The listing builds one solid part. Answer for the finished solid, in the listing's coordinates (mm). Coordinates: 2 decimals unless noted, no trailing zeros. One line per question, with ' | ' between items.
from build123d import *

# Parameters (mm, degrees)
SKETCH1_R               = 125
SKETCH1_R_2             = 32
BOSS_EXTRUDE1_DEPTH     = 4
CUT_EXTRUDE1_REACH      = 178.958
SKETCH2_R               = 4.5
CIRPATTERN2_COUNT       = 5
FILL_START              = -4
FILL_PATTERN1_OUTLINE_R = 4.5
FILL_PATTERN1_DEPTH     = 8
FILLET1_R               = 6.5


# Read off the part's stored shape, not the designer's step: Fill Pattern1
with BuildPart() as part:
    # Sketch1 → Boss-Extrude1 (new, symmetric)
    with BuildSketch(Plane.XY):
        Circle(SKETCH1_R)
        Circle(SKETCH1_R_2, mode=Mode.SUBTRACT)
    extrude(amount=BOSS_EXTRUDE1_DEPTH, both=True)

    # Sketch2 → Cut-Extrude1 (cut, up to next)
    with BuildSketch(Plane.XY.offset(4), mode=Mode.PRIVATE) as cut_extrude1_sk1:
        with BuildLine():
            ThreePointArc((-9.355894551, 30.601752191), (0, 32), (9.355894551, 30.601752191))
            Line((9.355894551, 30.601752191), (19.588904216, 64.07241865))
            ThreePointArc((19.588904216, 64.07241865), (0, 67), (-19.588904216, 64.07241865))
            Line((-19.588904216, 64.07241865), (-9.355894551, 30.601752191))
        make_face()
    cut_extrude1_tool1 = extrude(cut_extrude1_sk1.sketch, amount=-CUT_EXTRUDE1_REACH, mode=Mode.PRIVATE) & part.part
    # Sketch2 → Cut-Extrude1 (cut, up to next)
    with BuildSketch(Plane.XY.offset(4), mode=Mode.PRIVATE) as cut_extrude1_sk2:
        with Locations((-26.450336353, 36.405764747)):
            Circle(SKETCH2_R)
    cut_extrude1_tool2 = extrude(cut_extrude1_sk2.sketch, amount=-CUT_EXTRUDE1_REACH, mode=Mode.PRIVATE) & part.part
    cut_extrude1_1 = cut_extrude1_tool1.solids().sort_by_distance((0, 50.80907, 4))[0]
    add(cut_extrude1_1, mode=Mode.SUBTRACT)
    cut_extrude1_2 = cut_extrude1_tool2.solids().sort_by_distance((-26.450336, 36.405765, 4))[0]
    add(cut_extrude1_2, mode=Mode.SUBTRACT)
    cut_extrude1 = cut_extrude1_1 + cut_extrude1_2  # Cut-Extrude1 as one shape, for the pattern or mirror that repeats it

    # CirPattern2: Cut-Extrude1 ×5 about axis
    cirpattern2_axis = Axis((0, 0, 0), (0, 0, 1))
    for i in range(1, CIRPATTERN2_COUNT):
        add(cut_extrude1.rotate(cirpattern2_axis, i * 360 / CIRPATTERN2_COUNT), mode=Mode.SUBTRACT)

    # Fill Pattern1 outline → Fill Pattern1 (cut)
    with BuildSketch(Plane.XY.offset(FILL_START)):
        with Locations((-99.984772584, 1.745240337)):
            Circle(FILL_PATTERN1_OUTLINE_R)
        with Locations((-97.277590889, -23.174790656)):
            Circle(FILL_PATTERN1_OUTLINE_R)
        with Locations((-88.45810059, -46.638664341)):
            Circle(FILL_PATTERN1_OUTLINE_R)
        with Locations((-74.080462697, -67.172059239)):
            Circle(FILL_PATTERN1_OUTLINE_R)
        with Locations((-55.048077077, -83.484786633)):
            Circle(FILL_PATTERN1_OUTLINE_R)
        with Locations((-32.556818514, -94.551857867)):
            Circle(FILL_PATTERN1_OUTLINE_R)
        with Locations((-8.019895501, -99.677888152)):
            Circle(FILL_PATTERN1_OUTLINE_R)
        with Locations((17.020946849, -98.540790155)):
            Circle(FILL_PATTERN1_OUTLINE_R)
        with Locations((40.992300316, -91.212011924)):
            Circle(FILL_PATTERN1_OUTLINE_R)
        with Locations((62.387956603, -78.152047549)):
            Circle(FILL_PATTERN1_OUTLINE_R)
        with Locations((79.863547937, -60.181502622)):
            Circle(FILL_PATTERN1_OUTLINE_R)
        with Locations((92.321018643, -38.429532573)):
            Circle(FILL_PATTERN1_OUTLINE_R)
        with Locations((98.977620023, -14.262893677)):
            Circle(FILL_PATTERN1_OUTLINE_R)
        with Locations((99.415093329, 10.799935264)):
            Circle(FILL_PATTERN1_OUTLINE_R)
        with Locations((93.605950506, 35.184164534)):
            Circle(FILL_PATTERN1_OUTLINE_R)
        with Locations((81.915201361, 57.357643328)):
            Circle(FILL_PATTERN1_OUTLINE_R)
        with Locations((65.077418659, 75.927130427)):
            Circle(FILL_PATTERN1_OUTLINE_R)
        with Locations((44.150582211, 89.725836661)):
            Circle(FILL_PATTERN1_OUTLINE_R)
        with Locations((20.449602116, 97.886738569)):
            Circle(FILL_PATTERN1_OUTLINE_R)
        with Locations((-4.536301881, 99.897056672)):
            Circle(FILL_PATTERN1_OUTLINE_R)
        with Locations((-29.23717354, 95.63047529)):
            Circle(FILL_PATTERN1_OUTLINE_R)
        with Locations((-52.100966252, 85.355079421)):
            Circle(FILL_PATTERN1_OUTLINE_R)
        with Locations((-71.691063833, 69.716509979)):
            Circle(FILL_PATTERN1_OUTLINE_R)
        with Locations((-86.776548405, 49.697395796)):
            Circle(FILL_PATTERN1_OUTLINE_R)
        with Locations((-96.409543491, 26.555611442)):
            Circle(FILL_PATTERN1_OUTLINE_R)
    extrude(amount=FILL_PATTERN1_DEPTH, mode=Mode.SUBTRACT)

    # Fillet1
    fillet1_edges = [part.edges().sort_by_distance(p)[0] for p in [
        (19.588904216, 64.07241865, 0),
        (9.355894551, 30.601752191, 0),
        (-9.355894551, 30.601752191, 0),
        (-19.588904216, 64.07241865, 0),
        (-53.508579173, -40.321606551, 0),
        (-25.556336322, -19.258080741, 0),
        (-10.418180943, -30.256594419, 0),
        (-21.813066349, -63.349744565, 0),
        (21.813066349, -63.349744565, 0),
        (10.418180943, -30.256594419, 0),
        (25.556336322, -19.258080741, 0),
        (53.508579173, -40.321606551, 0),
        (66.989795575, 1.169311231, 0),
        (31.995126245, 0.558477006, 0),
        (26.212865417, 18.354445963, 0),
        (54.883186967, 38.429621236, 0),
        (-54.883186967, 38.429621236, 0),
        (-26.212865417, 18.354445963, 0),
        (-31.995126245, 0.558477006, 0),
        (-66.989795575, 1.169311231, 0),
    ]]
    fillet(fillet1_edges, radius=FILLET1_R)


solid = part.part
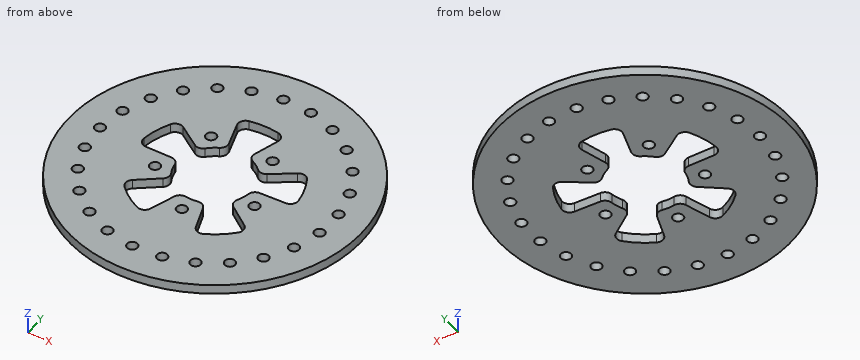
Item 1: Find the intervals of material crossed by line 1 (X direction, y = -11, z = -3.5); line 2 (Y direction, x = -49, z = -1.75); line 3 (X direction, y = 57.5, z = -3.5), in increasing order. Write a range as [from, to].
Taken from the geometry:
line 1: x = [-124.52, -46.23], [-39.36, -30.05], [30.05, 39.36], [46.23, 95.88], [102.08, 124.52] | line 2: y = [-115, -45.69], [-37.09, 0.86], [34.31, 82.09], [88.62, 115] | line 3: x = [-110.99, -17.58], [17.58, 77.42], [86.41, 110.99]
Item 2: Find section A-A, the plane z = 1. State how many separate pieces and enclosed holes the cut face has, plus the area to 3 significant figures.
Taken from the geometry:
separate pieces: 1 | enclosed holes: 31 | area: 38,900 mm2
Item 3: Each of these flat-tipped pins is pushed along its axis until it touches: pin 1 Ø5.5 at (x, y) = (-42.8, -13.91) entering from -Z; pin 2 Ø11.5 at (x, y) = (-8.02, -99.68) entering from -Z; pin 3 Ø3 at (y, z) = (93, -1.5) entering from -X; pin 4 Ø2 at (y, z) = (-49, -1.5) entering from +X. Where does it stop, or does it pass through?
Taken from the geometry:
pin 1: passes through | pin 2: stops at z = -4 | pin 3: stops at x = -85.16 | pin 4: stops at x = 115.42
